Input: dimensioned drawing with shaded views. Units: mm. Origin: part minimum x, y, z. A direction names the side the tool comes from. Round coordinates to 2 decimals unless told otherwise and drop trailing zeros. Order: outer loops, then holes, each group sorted by start corner. A loop starts at its lowest first (then second) coordinate and runs counter-clockwise, first axis right, second up. Notation, with made-up numbers: (4, -1) - (8, -1) arc R28 cw to (8, 36) - close; hole circle Ø9 at (72, -33). An arc over 180 degrees is marked (long way). Put each result on its own line as item: value. Start each with the question number.
(1) Pin query (flat end, axial travel): P1, Ø2, axis at y = 3, z = 10, coming from the -X side; P2, Ø4.5, axis at x = 40, y = 9.5, coming from the -Z side; P3, Ø4, axis at x = 35, z = 31.5, coming from the +Y side; P4, Ø5, axis at x = 24.5, y = 2.5, coming from the +Z side. Return the tip coordinate at first contact, or that it passes through.
(2) Section B-B (x = 49.5). Output: boundary loops of the cut face in (y, z).
(3) Section D-D (x = 29). Output: boundary loops of the cut face in (y, z), and give its area (3 significant figures).
(4) Section C-C (y = 9). Output: boundary loops of the cut face in (x, z).
(5) Section A-A (z = 21). Output: boundary loops of the cut face in (x, y).
(6) Pull-direction query (Z, two-part tool) for the marked faces 4, 5 and 6; classes: released by +Z, released by -Z, zero draft, split by the parting line, or undercut.
(7) Access query for the marked faces 1, 2 and 3. Directions: +Z, -Z, +X, -X, +Y, -Y. A direction counts if a zero-diameter tool reaches every point of the face in a straight line with its end or side. Return the directions, or none.
(8) Material intervals for L1, parallel to X at y = 3.5, z = 28; L2, parallel to Z at x = 39, y = 5.25; L3, parallel to Y at x = 24, z = 5, sorted ascending. Write a range as [from, to].
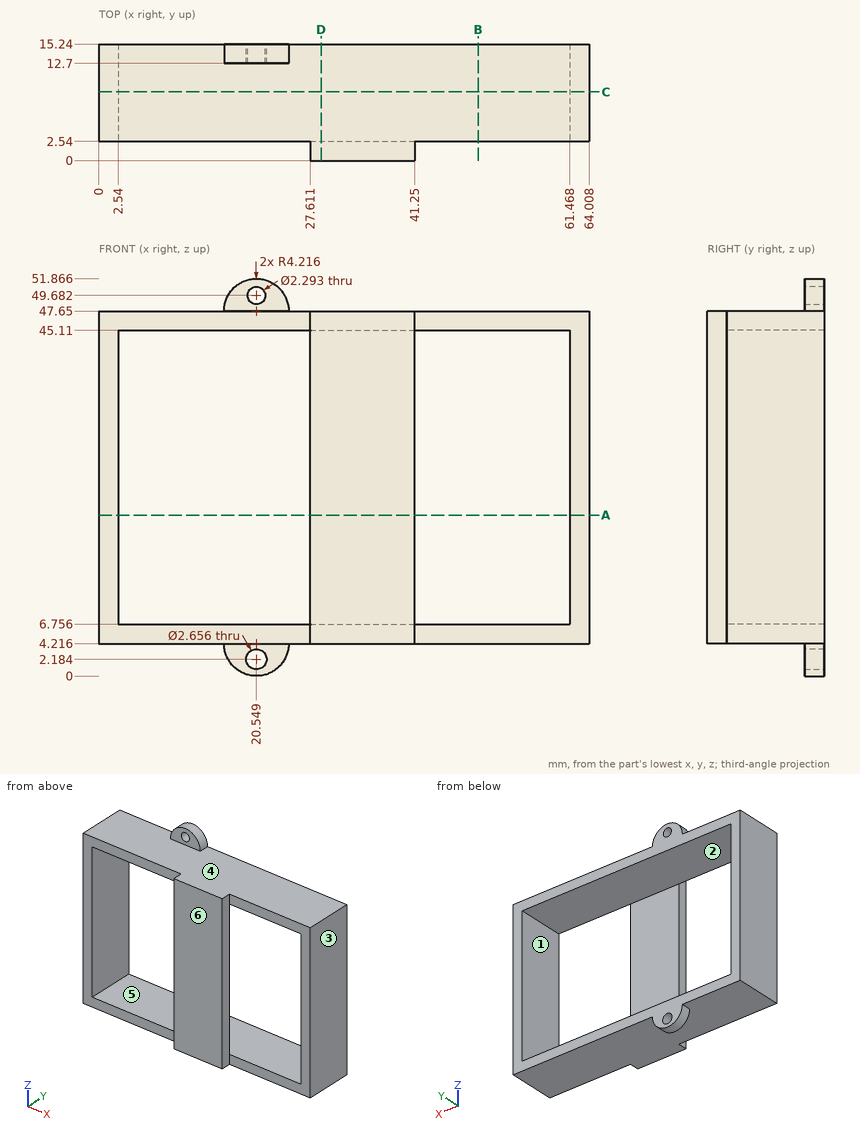
Checks:
1. P1: stops at x = 0
1. P2: stops at z = 4.22
1. P3: stops at y = 2.54
1. P4: stops at z = 47.65
2. outline: (2.54, 4.22) - (15.24, 4.22) - (15.24, 6.76) - (2.54, 6.76) - close; (2.54, 45.11) - (15.24, 45.11) - (15.24, 47.65) - (2.54, 47.65) - close
3. outline: (0, 4.22) - (15.24, 4.22) - (15.24, 6.76) - (2.54, 6.76) - (2.54, 45.11) - (15.24, 45.11) - (15.24, 47.65) - (0, 47.65) - close
3. area: 175 mm²
4. outline: (0, 4.22) - (64.01, 4.22) - (64.01, 47.65) - (0, 47.65) - close; hole (2.54, 6.76) - (61.47, 6.76) - (61.47, 45.11) - (2.54, 45.11) - close
5. outline: (0, 2.54) - (2.54, 2.54) - (2.54, 15.24) - (0, 15.24) - close; (27.61, 0) - (41.25, 0) - (41.25, 2.54) - (27.61, 2.54) - close; (61.47, 2.54) - (64.01, 2.54) - (64.01, 15.24) - (61.47, 15.24) - close
6. face 4: released by +Z
6. face 5: undercut
6. face 6: zero draft
7. face 1: +Y, -Y
7. face 2: +Y
7. face 3: +Z, -Z, +X, +Y, -Y
8. L1: x = [0, 2.54], [61.47, 64.01]
8. L2: z = [4.22, 6.76], [45.11, 47.65]
8. L3: y = [2.54, 15.24]
